Geometry check sheet. Reference: the model listing, model coordinates, mm. A direction names the side the tool comes from. Round coordinates to 2 decimals unless told otherwise and drop trailing zeros. Order: outer loops, then holes, each group sorted by start corner. A loop starts at its lowest first (then second) coordinate and runs counter-clockwise, first axis right, second up. Notation, with made-up numbers: (26.25, 64.5) - (37.25, 64.5) arc R22 ccw to (37.25, 79.5) - close; hole circle Ø11 at (66.25, 37.5). An arc over 180 degrees is marked (long way). Return JSON: item names as keys, results as strings. Group by question number.
Q1. Draft check along X on faces 1 (the flat face through (-41.179, 38, 117)), 2 (the flat face through (3, 76.901, 9)), 3 (the cylindrical face through (19.23, 89.3, 111.37)), 4 (the flat face through (28.671, 24, 9)). Enter one of: pulls with the +X half, pulls with the -X half, needs draft (parallel to the pull), parting line crosses it, or undercut.
Q2. Sectioned sample at A-A, the plane y = 83.5. Record the cut outline in (x, z).
Q3. Sectioned sample at C-C, the plane y = 25. Record the cut outline in (x, z).
Q4. Sectioned sample at B-B, the plane z = 41. Record the cut outline in (x, y), then the cut area to 3 significant figures.
Q5. Tool access check on faces 5 (the flat face through (-13, 94.932, 13)), 6 (the flat face through (-6.254, 85, 63)), 7 (the flat face through (25.496, 85.7, 62.6)). Record the directions out of +Z, -Z, +X, -X, +Y, -Y that give a thin tool (end or side, any length) a straight path to the whole face; none if there is none.
Q6. Gauge pin test, flat ends, axial feed: pin 1 Ø10 at (y, z) = (94.93, 114.3) entering from +X; pin 2 Ø24.5 at (y, z) = (85.5, 67) entering from -X; pin 3 Ø6.5 at (x, z) = (16.5, 80.5) entering from +Y; pin 4 Ø4 at (x, z) = (-7.5, 105) entering from -Y. Record the tip position at first contact, or that the pin passes through.
Q7. Material ranges on line 1 along X through (y, z) = (79, 97.5); line 2 along Z through (x, y) = (1, 66); line 3 along Y through (x, z) = (22, 50), recorded low to high.
Autodesk Inventor part; units mm, degrees
ref_plane "YZ Plane" through (0, 0, 0) normal (1, 0, 0) x (0, 1, 0)
ref_plane "XZ Plane" through (0, 0, 0) normal (0, 1, 0) x (-1, 0, 0)
ref_plane "XY Plane" through (0, 0, 0) normal (0, 0, 1) x (1, 0, 0)
sketch "front profile" plane through (0, 0, 0) normal (0, 0, 1) x (1, 0, 0)
  line L0 (47.7209, 56.8325) -> (47.7209, 18.7325)
  line L1 (-41.1791, 18.7325) -> (-41.1791, 56.8325)
  line L2 (25.4959, 107.6325) -> (25.4959, 76.9011)
  line L3 (12.7959, 76.9011) -> (-6.2541, 76.9011)
  line L4 (-18.9541, 76.9011) -> (-18.9541, 107.6325)
  line L5 (12.7959, 107.6325) -> (12.7959, 76.9011)
  line L6 (12.7959, 76.9011) -> (-6.2541, 76.9011)
  line L7 (-6.2541, 76.9011) -> (-6.2541, 107.6325)
  line L8 (25.4959, 76.9011) -> (47.7209, 56.8325)
  line L9 (-18.9541, 76.9011) -> (-41.1791, 56.8325)
  line L10 (28.6709, 18.7325) -> (28.6709, 30.003)
  line L11 (-22.1291, 30.003) -> (-22.1291, 18.7325)
  arc A0 (28.6709, 30.003) -> (-22.1291, 30.003) centre (3.2709, 30.003) ccw
  line L12 (-18.9541, 107.6325) -> (-6.2541, 107.6325)
  line L13 (12.7959, 107.6325) -> (25.4959, 107.6325)
  line L14 (47.7209, 18.7325) -> (28.6709, 18.7325)
  line L15 (-22.1291, 18.7325) -> (-41.1791, 18.7325)
  line L16 (-18.9541, 107.6325) -> (-6.2541, 107.6325)
  line L17 (12.7959, 107.6325) -> (25.4959, 107.6325)
  point P0 (-6.2541, 92.2668)
  point P1 (-12.6041, 107.6325)
  point P2 (19.1459, 107.6325)
  dimension "d2" = 88.9
  dimension "d9" = 22.225
  dimension "d10" = 22.225
  dimension "d11" = 12.7
  dimension "d12" = 12.7
  dimension "d14" = 38.1
  dimension "d15" = 38.1
  dimension "d17" = 19.05
  dimension "d18" = 19.05
  dimension "d32" = 88.9
  dimension "d33" = 88.9
  dimension "d34" = 25.4
  dimension "d36" = 47.919
  dimension "d37" = 47.919
  dimension "d39" = 58.1686
  dimension "d40" = 88.9
  dimension "d43" = 11.2705
extrude "front profile Extrusion" add sketch "front profile" along normal blind 127
sketch "side profile" plane through (25.4959, 76.9011, 0) normal (1, 0, 0) x (0, 0, -1)
  line L0 (0, -20.0686) -> (0, -58.1686)
  line L1 (-127, 30.7314) -> (0, 30.7314)
  line L2 (0, 30.7314) -> (0, -58.1686)
  line L3 (0, -58.1686) -> (-127, -58.1686)
  line L4 (-127, -58.1686) -> (-127, 18.0314)
  line L5 (-25.4, 18.0314) -> (-25.4, 9.0465)
  line L6 (-25.4, 9.0465) -> (-101.6, 9.0465)
  line L7 (-101.6, 9.0465) -> (-101.6, 18.0314)
  line L8 (0, 0) -> (-127, 0)
  line L9 (0, -58.1686) -> (-127, -58.1686)
  line L10 (-107.95, 0) -> (-19.05, 0)
  line L11 (-19.05, 0) -> (-19.05, -58.1686)
  line L12 (-19.05, -58.1686) -> (-107.95, -58.1686)
  line L13 (-107.95, -58.1686) -> (-107.95, 0)
  circle A0 centre (-114.3, 18.0314) radius 6.35
  arc A1 (-101.6, 18.0314) -> (-127, 18.0314) centre (-114.3, 18.0314) ccw
  line L14 (0, 30.7314) -> (-127, 30.7314)
  line L15 (-25.4, 18.0314) -> (0, 18.0314)
  point P0 (0, -76.9011)
  point P1 (-114.3, 30.7314)
  point P2 (-107.95, -58.1686)
  point P3 (-19.05, -58.1686)
  point P4 (-19.05, 0)
  dimension "d23" = 25.4
  dimension "d24" = 19.05
  dimension "d25" = 19.05
  dimension "d26" = 12.7
  dimension "d27" = 12.7
  dimension "d35" = 127
  dimension "d45" = 12.7
  dimension "d46" = 30.7314
  dimension "d47" = 19.05
  dimension "d48" = 88.9
  dimension "d49" = 19.05
  dimension "d50" = 88.9
  dimension "d51" = 107.95
  dimension "d52" = 0
  dimension "d53" = 114.3
  dimension "d54" = 21.6849
extrude "side profile extrusion" cut sketch "side profile" along normal through all both and the other way through all contours L3 L13 L8 L11 | L15 L5 L6 L7 A1 L1 L2 | A0
fillet "Front Fillet" radius 12.7 2 edges at (19.1459, 107.6325, 127) (-12.6041, 107.6325, 127)
equation "\"d10\" = d9"
equation "\"d15\" = d14"
equation "\"d17\" = d16"
equation "\"d37\" = d36"
equation "\"d25\" = d24"
properties part number "ASN4-4-BK" material "Iron, Cast"
Reply:
{
 "1": {"face 1": "pulls with the -X half", "face 2": "undercut", "face 3": "needs draft", "face 4": "undercut"},
 "2": {"outline": "(-18.95, 0) - (-6.25, 0) - (-6.25, 127) - (-18.95, 127) - close; (12.8, 0) - (25.5, 0) - (25.5, 127) - (12.8, 127) - close"},
 "3": {"outline": "(-41.18, 0) - (-22.13, 0) - (-22.13, 19.05) - (-41.18, 19.05) - close; (-41.18, 107.95) - (-22.13, 107.95) - (-22.13, 127) - (-41.18, 127) - close; (28.67, 0) - (47.72, 0) - (47.72, 19.05) - (28.67, 19.05) - close; (28.67, 107.95) - (47.72, 107.95) - (47.72, 127) - (28.67, 127) - close"},
 "4": {"outline": "(-18.95, 76.9) - (-6.25, 76.9) - (-6.25, 85.95) - (-18.95, 85.95) - close; (12.8, 76.9) - (25.5, 76.9) - (25.5, 85.95) - (12.8, 85.95) - close", "area": "230 mm^2"},
 "5": {"face 5": "-Z, +X, -X, +Y", "face 6": "+Z, -Z, +Y", "face 7": "+Z, -Z, +X, +Y"},
 "6": {"pin 1": "through", "pin 2": "x = -18.95", "pin 3": "y = 85.95", "pin 4": "y = 76.9"},
 "7": {"line 1": "-18.95 to -6.25, 12.8 to 25.5", "line 2": "0 to 19.05, 107.95 to 127", "line 3": "76.9 to 85.95"}
}
